Check sheet for the modelled part. Datum: model origin and axes. Units: mm. A direction names the side the tool comes from. Give positions to 0.01 mm unless a question says otherwise; leave off trailing zeros. Order: outer loops, then holes, each group sorted by start corner. A loop starts at its lowest first (then second) coordinate and runs counter-clockwise, first axis right, second up.
Item 1: Gauge pin test, flat ends, axial feed: P1, Ø12.5, axis at y = -35.5, z = -15, coming from the +X side; P2, Ø1.5, axis at x = -7.5, y = -18.5, coming from the +Z side; P3, Ø5, axis at x = -9, y = -43.5, coming from the +Z side. Record the tip position at first contact, or that the pin passes through.
Item 2: Sectioned sample at B-B on y = -9. Record the boundary of the cut face in (x, z).
Item 3: Material ranges on line 1 along Z through (x, y) = (0, -38); line 2 along X through (y, z) = (-47.5, -18); line 3 along Y through (x, z) = (34, -18.5), recorded low to high.
Item 4: Sectioned sample at A-A on x = 0. Record the boundary of the cut face in (y, z), and give its area (3 significant figures).
Item 5: Access from +Z, -Z, +X, -X, +Y, -Y to the whole of each face (thin tool, end or side, straight path). Record for faces 1 (the flat face through (37, -38, -50.653)), 2 (the flat face through (64, -38, -38.381)), 3 (the flat face through (101.44, -32, -45)), 4 (the flat face through (101.6, -13, -45)), 5 (the flat face through (-25.4, -25, -25)).
Item 6: Sectioned sample at D-D on x = 80.5. Record the boundary of the cut face in (y, z), and give its area (3 significant figures).
Item 7: Sectioned sample at C-C on z = -10. Record the boundary of the cut face in (x, y).
from build123d import *

# Parameters (mm, degrees)
F0_R     = 12.7
F1_DEPTH = 25.4
F2_R     = 12.7
F3_DEPTH = 25.4
F4_R     = 12.7


with BuildPart() as f1:
    # F0 (on Front) → F1 (new body)
    with BuildSketch(Plane.XZ):
        with BuildLine():
            Line((101.6, -38.1), (14.244434, 21.029886))
            ThreePointArc((14.244434, 21.029886), (-11.90276, 22.438456), (-25.4, 0))
            Line((-25.4, 0), (-25.4, -50.8))
            Line((-25.4, -50.8), (101.6, -50.8))
            Line((101.6, -50.8), (101.6, -38.1))
        make_face()
        Circle(F0_R, mode=Mode.SUBTRACT)
    extrude(amount=F1_DEPTH)

    # F2 (on face) → F3 (join)
    with BuildSketch(Plane.XZ.offset(25.4)):
        with BuildLine():
            Line((25.4, -38.380738), (25.4, 0))
            ThreePointArc((25.4, 0), (22.438456, 11.90276), (14.244434, 21.029886))
            ThreePointArc((14.244434, 21.029886), (-11.90276, 22.438456), (-25.4, 0))
            Line((-25.4, 0), (-25.4, -50.652947))
            Line((-25.4, -50.652947), (101.439578, -50.652947))
            Line((101.439578, -50.652947), (101.439578, -38.380738))
            Line((101.439578, -38.380738), (25.4, -38.380738))
        make_face()
        Circle(F2_R, mode=Mode.SUBTRACT)
    extrude(amount=F3_DEPTH)

    # F4
    f4_edges = [f1.edges().sort_by_distance(p)[0] for p in [
        (101.439578, -50.8, -44.516843),
    ]]
    fillet(f4_edges, radius=F4_R)


solid = f1.part
Report:
1. P1: stops at x = 25.4
1. P2: stops at z = 24.49
1. P3: stops at z = 24.55
2. outline: (-25.4, -50.8) - (101.6, -50.8) - (101.6, -38.1) - (14.24, 21.03) arc R25.4 ccw to (-25.4, 0) - close; hole circle Ø25.4 at (0, 0)
3. line 1: z = -50.65 to -12.7, 12.7 to 25.4
3. line 2: x = -25.4 to 25.4
3. line 3: y = -25.4 to 0
4. outline: (-50.8, -50.65) - (-25.4, -50.65) - (-25.4, -50.8) - (0, -50.8) - (0, -12.7) - (-50.8, -12.7) - close; (-50.8, 12.7) - (0, 12.7) - (0, 25.4) - (-50.8, 25.4) - close
4. area: 2,580 mm2
5. face 1: -Z, +X, -X, -Y
5. face 2: +Z, +X, -Y
5. face 3: +Z, -Z, +X, -Y
5. face 4: +Z, -Z, +X, +Y, -Y
5. face 5: +Z, -Z, -X, +Y, -Y
6. outline: (-50.8, -50.65) - (-25.4, -50.65) - (-25.4, -50.8) - (0, -50.8) - (0, -23.82) - (-25.4, -23.82) - (-25.4, -38.38) - (-50.8, -38.38) - close
6. area: 997 mm2
7. outline: (-25.4, -50.8) - (-7.83, -50.8) - (-7.83, 0) - (-25.4, 0) - close; (7.83, -50.8) - (25.4, -50.8) - (25.4, -25.4) - (60.09, -25.4) - (60.09, 0) - (7.83, 0) - close
